```python
from build123d import *

# Parameters (mm, degrees)
SKETCH1_W           = 20
SKETCH1_H           = 20
BOSS_EXTRUDE1_DEPTH = 6
SKETCH2_W           = 6.8
SKETCH2_H           = 20
BOSS_EXTRUDE2_DEPTH = 6
SKETCH3_W           = 7
SKETCH3_H           = 20
BOSS_EXTRUDE3_DEPTH = 15
CHAMFER1_SIZE       = 6
SKETCH4_R           = 3
CUT_EXTRUDE1_DEPTH  = 10
SKETCH5_W           = 20
SKETCH5_H           = 20
BOSS_EXTRUDE4_DEPTH = 18
CUT_EXTRUDE2_DEPTH  = 2
SKETCH7_R           = 2.8
CUT_EXTRUDE3_DEPTH  = 20
CUT_EXTRUDE4_DEPTH  = 6


with BuildPart() as part:
    # Sketch1 → Boss-Extrude1 (new body)
    with BuildSketch(Plane(origin=(0, 0, 0), x_dir=(1, 0, 0), z_dir=(0, 1, 0))):
        Rectangle(SKETCH1_W, SKETCH1_H)
    extrude(amount=BOSS_EXTRUDE1_DEPTH)

    # Sketch2 → Boss-Extrude2 (add)
    with BuildSketch(Plane(origin=(0, 6, 0), x_dir=(1, 0, 0), z_dir=(0, 1, 0))):
        with Locations((6.6, 0)):
            Rectangle(SKETCH2_W, SKETCH2_H)
    extrude(amount=BOSS_EXTRUDE2_DEPTH)

    # Sketch3 → Boss-Extrude3 (add)
    with BuildSketch(Plane(origin=(0, 6, 0), x_dir=(1, 0, 0), z_dir=(0, 1, 0))):
        with Locations((-6.5, 0)):
            Rectangle(SKETCH3_W, SKETCH3_H)
    extrude(amount=BOSS_EXTRUDE3_DEPTH)

    # Chamfer1
    chamfer1_edges = [part.edges().sort_by_distance(p)[0] for p in [
        (-10, 21, 0),
    ]]
    chamfer(chamfer1_edges, length=CHAMFER1_SIZE)

    # Sketch4 → Cut-Extrude1 (cut)
    with BuildSketch(Plane(origin=(-12.5, 12.5, 0), x_dir=(0, 0, 1), z_dir=(-0.7071067811865489, 0.7071067811865462, 0))):
        with Locations(Location((0, 7.432512212, 0), (0, 0, 270))):
            Circle(SKETCH4_R)
    extrude(amount=-CUT_EXTRUDE1_DEPTH, mode=Mode.SUBTRACT)

    # Sketch5 → Boss-Extrude4 (add)
    with BuildSketch(Plane.XZ):
        Rectangle(SKETCH5_W, SKETCH5_H)
    extrude(amount=BOSS_EXTRUDE4_DEPTH)

    # Sketch6 → Cut-Extrude2 (cut)
    with BuildSketch(Plane(origin=(-12.5, 12.5, 0), x_dir=(0, 0, 1), z_dir=(-0.7071067811865489, 0.7071067811865462, 0))):
        Polygon((0, 13.8411002), (-5.55, 10.636806206), (-5.55, 4.228218218), (0, 1.023924224), (5.55, 4.228218218), (5.55, 10.636806206), align=None)
    extrude(amount=-CUT_EXTRUDE2_DEPTH, mode=Mode.SUBTRACT)

    # Sketch7 → Cut-Extrude3 (cut)
    with BuildSketch(Plane(origin=(0, -18, 0), x_dir=(-1, 0, 0), z_dir=(0, -1, 0))):
        with Locations(Location((0, 0, 0), (0, 0, 90))):
            Circle(SKETCH7_R)
    extrude(amount=-CUT_EXTRUDE3_DEPTH, mode=Mode.SUBTRACT)

    # Sketch8 → Cut-Extrude4 (cut)
    with BuildSketch(Plane(origin=(0, -18, 0), x_dir=(-1, 0, 0), z_dir=(0, -1, 0))):
        Polygon((5.038618856, -2.935243322), (5.061304711, 2.895950268), (0.022685855, 5.83119359), (-5.038618856, 2.935243322), (-5.061304711, -2.895950268), (-0.022685855, -5.83119359), align=None)
    extrude(amount=-CUT_EXTRUDE4_DEPTH, mode=Mode.SUBTRACT)


solid = part.part
```
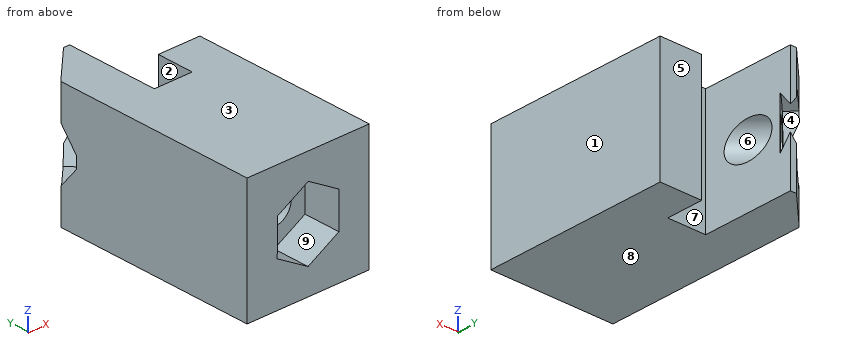
Build history of the part. All positions in model axes, mm. Face numbers are marked on the shaded views. A direction names the side the tool comes from. Coordinates: 2 decimals unless noted, no trailing zeros. Order: outer loops, then holes, each group sorted by start corner. A loop starts at its lowest first (then second) coordinate and runs counter-clockwise, first axis right, second up.
Item 1: Mould opens along Z. For the marked faces 6, 7, 8 and 9 say: released by +Z, released by -Z, zero draft, split by the parting line, or undercut.
Filled in:
face 6: undercut
face 7: zero draft
face 8: released by -Z
face 9: undercut
Item 2: Saw through at D-D on x = -0.75. List the corners of the cut face in (y, z).
Filled in:
outline: (-18, -10) - (6, -10) - (6, 10) - (-18, 10) - (-18, 5.39) - (-12, 5.39) - (-12, 2.7) - (2, 2.7) - (2, -2.7) - (-12, -2.7) - (-12, -5.41) - (-18, -5.41) - close
Item 3: Drill centre lines: L1, parallel to X at y = -6.5, z = 0; L2, parallel to X at y = 8, z = 1.5; L3, parallel to Y at x = 6.75, z = 5.5. Where is each one in solid material? Low to high.
Filled in:
L1: x = -10 to -2.8, 2.8 to 10
L2: x = -10 to -3, 3.2 to 10
L3: y = -18 to 12
Item 4: Saw through at A-A on z = 0. List the corners of the cut face in (x, y), then the cut area to 3 significant figures.
Filled in:
outline: (-10, -18) - (-5.05, -18) - (-5.05, -12) - (-2.8, -12) - (-2.8, 2) - (2.8, 2) - (2.8, -12) - (5.05, -12) - (5.05, -18) - (10, -18) - (10, 12) - (3.2, 12) - (3.2, 6) - (-3, 6) - (-3, 9.27) - (-7.95, 14.22) - (-10, 12.17) - close; (-3.71, 18.46) - (-3, 17.75) - (-3, 19.17) - close
area: 425 mm2
Item 5: Saw through at B-B on y = -9. List the corners of the cut face in (x, z), then the cut area to 3 significant figures.
Filled in:
outline: (-10, -10) - (10, -10) - (10, 10) - (-10, 10) - close; hole circle Ø5.6 at (0, 0)
area: 375 mm2
Item 6: Drop flat-ended pins along their axis: pin 1 Ø5.5 at (x, z) = (6, -3) entering from +Y; pin 2 Ø5 at (x, z) = (0, 4) entering from +Y; pin 3 Ø6.5 at (x, z) = (0, 0) entering from -Y. Give the stop position or say it passes through.
Filled in:
pin 1: stops at y = 12
pin 2: stops at y = 6
pin 3: stops at y = -12
Item 7: Tool access for the marked faces 1, 2, 3, 4 and 5: list every direction of +Z, -Z, +X, -X, +Y, -Y with a clear straight run to the whole face (end or side of a thin tool).
Filled in:
face 1: +Z, -Z, +X, +Y, -Y
face 2: +Z, -Z, +Y
face 3: +Z, +X, -X, +Y, -Y
face 4: +Y
face 5: +Z, -Z, +X, +Y
Item 8: Saw through at C-C on z = 6.75. List the corners of the cut face in (x, y), then the cut area to 3 significant figures.
Filled in:
outline: (-10, -18) - (10, -18) - (10, 12) - (3.2, 12) - (3.2, 6) - (-3, 6) - (-3, 21) - (-4, 21) - (-10, 15) - close
area: 608 mm2
